Source: CAD feature listing. Evaluate the final solid. Frame: model axes, mm. Coordinates: 2 decimals unless noted, no trailing zeros. Loops run counter-clockwise (first coordinate to the right, second up) from the corner with the lowest first, then second, coordinate; pieces in that order, holes last.
```python
from build123d import *

# Parameters (mm, degrees)
RETAINING_PLATE_START               = 33.8
RETAINING_PLATE_DEPTH               = 1.8
PLUNGERS_AND_M2P5_SCREWS_DEPTH      = 117.372677206
PLUNGERS_AND_M2P5_SCREWS_DEPTH_BACK = 117.372677206
SKETCH_2_R                          = 3.6
SKETCH_2_R_2                        = 1.4


with BuildPart() as part:
    # 草图1 → Retaining_plate (new body)
    with BuildSketch(Plane.XY.offset(RETAINING_PLATE_START)):
        with BuildLine():
            Line((52, 45.5), (90, 45.5))
            ThreePointArc((90, 45.5), (90.707106781, 45.792893219), (91, 46.5))
            Line((91, 46.5), (91, 62.2))
            ThreePointArc((91, 62.2), (90.707106781, 62.907106781), (90, 63.2))
            Line((90, 63.2), (52, 63.2))
            ThreePointArc((52, 63.2), (51.292893219, 62.907106781), (51, 62.2))
            Line((51, 62.2), (51, 46.5))
            ThreePointArc((51, 46.5), (51.292893219, 45.792893219), (52, 45.5))
        make_face()
    extrude(amount=RETAINING_PLATE_DEPTH)

    # 草图2 → Plungers_and_M2p5_screws (cut, two sides: drawn at the far end of the back side and taken through both)
    with BuildSketch(Plane.XY.offset(-PLUNGERS_AND_M2P5_SCREWS_DEPTH_BACK)):
        with Locations((59, 54.355)):
            Circle(SKETCH_2_R)
        with Locations((71, 54.355)):
            Circle(SKETCH_2_R)
        with Locations((83, 54.355)):
            Circle(SKETCH_2_R)
        with Locations((54, 48.5)):
            Circle(SKETCH_2_R_2)
        with Locations((88, 60.2)):
            Circle(SKETCH_2_R_2)
    extrude(amount=PLUNGERS_AND_M2P5_SCREWS_DEPTH + PLUNGERS_AND_M2P5_SCREWS_DEPTH_BACK, mode=Mode.SUBTRACT)


solid = part.part
```
Q1. Draft query along Y for faces 1 (the flat face through (71, 45.5, 35)), 2 (the flat face through (51, 54, 35)), 3 (the cylindrical face through (87.82, 61.59, 34.69)). Return one class per face: released by +Y, released by -Y, zero draft, split by the parting line, or undercut.
Q2. Section query C-C on z = 34.2. Return the cut outline in (x, y) (3 decimals), then the cut area to 3 significant figures.
Q3. Section query D-D on y = 56.5. Return the cut outline in (x, z), then the cut area to 3 significant figures.
Q4. Material intervals for line 1 along X through (y, z) = (54.5, 34.45); line 2 along X through (y, z) = (48.5, 34.6); line 3 along Y through (x, z) = (88, 35.15), sorted ascending.
Q5. Section query B-B on x = 83. Return the cut outline in (y, z) (3 decimals).
Q6. Section query A-A on y = 60.2. Return the cut outline in (x, z), then the cut area to 3 significant figures.
Resolved:
1. face 1: released by -Y
1. face 2: zero draft
1. face 3: undercut
2. outline: (51, 46.5) arc R1 ccw to (52, 45.5) - (90, 45.5) arc R1 ccw to (91, 46.5) - (91, 62.2) arc R1 ccw to (90, 63.2) - (52, 63.2) arc R1 ccw to (51, 62.2) - close; hole circle Ø2.8 at (54, 48.5); hole circle Ø7.2 at (59, 54.355); hole circle Ø7.2 at (71, 54.355); hole circle Ø7.2 at (83, 54.355); hole circle Ø2.8 at (88, 60.2)
2. area: 573 mm2
3. outline: (51, 33.8) - (56.11, 33.8) - (56.11, 35.6) - (51, 35.6) - close; (61.89, 33.8) - (68.11, 33.8) - (68.11, 35.6) - (61.89, 35.6) - close; (73.89, 33.8) - (80.11, 33.8) - (80.11, 35.6) - (73.89, 35.6) - close; (85.89, 33.8) - (91, 33.8) - (91, 35.6) - (85.89, 35.6) - close
3. area: 40.8 mm2
4. line 1: x = 51 to 55.4, 62.6 to 67.4, 74.6 to 79.4, 86.6 to 91
4. line 2: x = 51 to 52.6, 55.4 to 91
4. line 3: y = 45.5 to 58.8, 61.6 to 63.2
5. outline: (45.5, 33.8) - (50.755, 33.8) - (50.755, 35.6) - (45.5, 35.6) - close; (57.955, 33.8) - (63.2, 33.8) - (63.2, 35.6) - (57.955, 35.6) - close
6. outline: (51, 33.8) - (86.6, 33.8) - (86.6, 35.6) - (51, 35.6) - close; (89.4, 33.8) - (91, 33.8) - (91, 35.6) - (89.4, 35.6) - close
6. area: 67.0 mm2
